```python
from build123d import *

# Parameters (mm, degrees)
SKETCH1_R               = 7
SKETCH1_R_2             = 4.05
BOSS_EXTRUDE1_DEPTH     = 15
BOSS_EXTRUDE2_START     = -15
SKETCH1_3_R             = 7
SKETCH1_3_R_2           = 4.05
SKETCH1_3_R_3           = 1.7
BOSS_EXTRUDE2_DEPTH     = 15
CUT_EXTRUDE1_DEPTH      = 18.972200756
CUT_EXTRUDE1_DEPTH_BACK = 18.972200756
SKETCH2_R               = 1.5


with BuildPart() as part:
    # Sketch1 → Boss-Extrude1 (new body)
    with BuildSketch(Plane(origin=(0, 0, 0), x_dir=(1, 0, 0), z_dir=(0, 1, 0))):
        with Locations(Location((0, 0, 0), (0, 0, 270))):
            Circle(SKETCH1_R)
        with Locations(Location((0, 0, 0), (0, 0, 270))):
            Circle(SKETCH1_R_2, mode=Mode.SUBTRACT)
    extrude(amount=BOSS_EXTRUDE1_DEPTH)

    # Sketch1_3 → Boss-Extrude2 (add)
    # profile 1 of 2: a face of its own
    with BuildSketch(Plane(origin=(0, 0, 0), x_dir=(1, 0, 0), z_dir=(0, 1, 0)).offset(BOSS_EXTRUDE2_START)):
        with Locations(Location((0, 0, 0), (0, 0, 270))):
            Circle(SKETCH1_3_R)
        with Locations(Location((0, 0, 0), (0, 0, 270))):
            Circle(SKETCH1_3_R_2, mode=Mode.SUBTRACT)
    # profile 2 of 2: a face of its own
    with BuildSketch(Plane(origin=(0, 0, 0), x_dir=(1, 0, 0), z_dir=(0, 1, 0)).offset(BOSS_EXTRUDE2_START)):
        with Locations(Location((0, 0, 0), (0, 0, 270))):
            Circle(SKETCH1_3_R_2)
        with Locations(Location((0, 0, 0), (0, 0, 270))):
            Circle(SKETCH1_3_R_3, mode=Mode.SUBTRACT)
    extrude(amount=BOSS_EXTRUDE2_DEPTH)

    # Sketch2 → Cut-Extrude1 (cut, two sides: drawn at the far end of the back side and taken through both)
    with BuildSketch(Plane.XY.offset(-CUT_EXTRUDE1_DEPTH_BACK)):
        with Locations((0, 8)):
            Circle(SKETCH2_R)
        with Locations((0, -8)):
            Circle(SKETCH2_R)
    extrude(amount=CUT_EXTRUDE1_DEPTH + CUT_EXTRUDE1_DEPTH_BACK, mode=Mode.SUBTRACT)


solid = part.part
```
For this review, take the finished solid that the model builds, in its own axes (mm). A direction names the side the tool comes from. Coordinates: 2 decimals unless noted, no trailing zeros. Write each loop counter-clockwise with the first axis right and the second up, starting at its lowest first coordinate (ties: lowest second). Pieces come first, ordered by that corner, then holes.
(1) For pin 1 Ø2 at (x, y) = (2.5, 3.5) entering from +Z; pin 2 Ø5 at (x, z) = (0, 0) entering from +Y; pin 3 Ø2 at (x, y) = (4, -2.5) entering from +Z, all flat-tipped, find the tip position at first contact; note any pin that passes through.
(2) Tool access review of faces 1 (the face through (-2.681, -0.21, 6.466)), 2 (the face through (0, 0, 2)): name each direction out of +Z, -Z, +X, -X, +Y, -Y from which nothing blocks a thin tool from reaching the whole face with its end or side.
(3) Add section C-C on z = 0. Give the boundary of the cut face in (x, y).
(4) Add section B-B on y = 8. Give the boundary of the cut face in (x, z), then the cut area to 3 significant figures.
(5) Wall thickness on probe 1 along Y at (x, z) = (0, 5); probe 2 along Y at (x, z) = (-0.75, -6); probe 3 along Z at (x, y) = (0, -4.25): over which ranges is each line inside the solid? List them lowest first.
(6) Add section D-D on z = -3. Give the boundary of the cut face in (x, y), then the cut area to 3 significant figures.
(7) Add section A-A on x = 0. Give the boundary of the cut face in (y, z).
(8) The part is to be moulded in two halves that separate along Y. For faces 3 (the face through (-1.5, -15, 1.5)), 4 (the face through (-1.5, 8.07, 5.36)), 5 (the face through (1.386, 7.425, -5.405)), 6 (the face through (-1.66, -7.6, -0.37)), say which applies: +Y half, -Y half, draft (parallel to the pull), parting line (faces both ways), or undercut.
Answer sheet:
1. pin 1: stops at z = 6.84
1. pin 2: stops at y = 0
1. pin 3: stops at z = 6.32
2. face 1: +Y, -Y
2. face 2: +Y
3. outline: (-7, -15) - (-1.7, -15) - (-1.7, 0) - (-4.05, 0) - (-4.05, 15) - (-7, 15) - close; (1.7, -15) - (7, -15) - (7, 15) - (4.05, 15) - (4.05, 0) - (1.7, 0) - close
4. outline: (-1.5, -6.84) - (-1.5, -3.76) arc R4.05 cw to (-1.5, 3.76) - (-1.5, 6.84) arc R7 ccw to start; (1.5, -6.84) arc R7 ccw to (1.5, 6.84) - (1.5, 3.76) arc R4.05 cw to (1.5, -3.76) - close
4. area: 84.5 mm2
5. probe 1: y = -15 to -9.5, -6.5 to 6.5, 9.5 to 15
5. probe 2: y = -15 to -9.3, -6.7 to 6.7, 9.3 to 15
5. probe 3: z = -7 to -1.7, 1.7 to 7
6. outline: (-6.32, -15) - (6.32, -15) - (6.32, 15) - (2.72, 15) - (2.72, 0) - (-2.72, 0) - (-2.72, 15) - (-6.32, 15) - close; hole circle Ø3 at (0, -8)
6. area: 291 mm2
7. outline: (-15, -7) - (-9.5, -7) - (-9.5, -1.7) - (-15, -1.7) - close; (-15, 1.7) - (-9.5, 1.7) - (-9.5, 7) - (-15, 7) - close; (-6.5, -7) - (6.5, -7) - (6.5, -4.05) - (0, -4.05) - (0, -1.7) - (-6.5, -1.7) - close; (-6.5, 1.7) - (0, 1.7) - (0, 4.05) - (6.5, 4.05) - (6.5, 7) - (-6.5, 7) - close; (9.5, -7) - (15, -7) - (15, -4.05) - (9.5, -4.05) - close; (9.5, 4.05) - (15, 4.05) - (15, 7) - (9.5, 7) - close
8. face 3: -Y half
8. face 4: undercut
8. face 5: undercut
8. face 6: draft
